The listing builds one solid part. Answer for the finished solid, in the listing's coordinates (mm). A direction names the side the tool comes from. Give positions to 0.01 mm unless a question says otherwise; leave off trailing zeros. Loops run counter-clockwise (first coordinate to the right, second up) from the corner with the lowest first, then second, coordinate; pieces in that order, holes last. Notation, with made-up numbers: (42, 49.5) - (73, 49.5) arc R27 ccw to (73, 83.5) - close; hole circle Ø2 at (56.25, -35). An arc over 180 degrees is marked (long way). Answer as CSV lines item,"result". Start each with the question number.
1) A cutting plane is placed at D-D (z = 49). Determine the outline of the cut face in (x, y) (3 decimals).
2) Find the intervals of material crossed by line 1 along Z through (x, y) = (11, -15.5) (3 decimals); line 2 along X through (y, z) = (10.5, 45.5); line 3 along Z through (x, y) = (-10, 4.5) (3 decimals), in increasing order.
3) For a pull along Z with two mould halves and no side action, classify faces 1 (the face through (-9, -9, 82.6)), 2 (the face through (19.98, -0.88, 69.71)), 3 (the face through (-9, 4, 25.425)) as pulls with the +Z half, pulls with the -Z half, needs draft (parallel to the pull), parting line crosses it, or undercut.
4) For faces 4 (the face through (0, 11.604, 42)), 5 (the face through (11.923, 3.755, 91.219)), 6 (the face through (11.923, 3.755, -8.381)), 7 (the face through (2.381, 10, 42)), determine the directions among +Z, -Z, +X, -X, +Y, -Y from which every point of the face is accessible in a straight line to the end or side of a thin tool.
5) Flat-ended cylindrical pins translate along their axes: pin 1 (1 mm diameter, centred on x = -10.5, y = 8, fed in from -Z); pin 2 (10 mm diameter, centred on x = -11.5, z = 78, fed in from +Y); pin 3 (6 mm diameter, centred on x = 13, y = -16, fed in from +Z). Find the tip coordinate at first contact, or state that the pin passes through.
6) A cutting plane is placed at C-C (x = 0). Determine the outline of the cut face in (y, z) (3 decimals), and give its area (3 significant figures).
7) A cutting plane is placed at A-A (y = 0). Determine the outline of the cut face in (x, z) (3 decimals).
8) A cutting plane is placed at B-B (x = 15.5). Determine the outline of the cut face in (y, z) (3 decimals).
```python
from build123d import *

# Parameters (mm, degrees)
SKETCH1_R           = 12.5
BOSS_EXTRUDE1_DEPTH = 17
SKETCH2_R           = 20
BOSS_EXTRUDE2_DEPTH = 25.425
SKETCH3_R           = 9.525
BOSS_EXTRUDE3_DEPTH = 31.75
SKETCH9_W           = 4.7625
SKETCH9_H           = 2.38125
BOSS_EXTRUDE6_DEPTH = 31.75
SKETCH4_R           = 20
BOSS_EXTRUDE4_DEPTH = 25.425
BOSS_EXTRUDE5_START = 17
SKETCH5_R           = 12.5
BOSS_EXTRUDE5_DEPTH = 17


with BuildPart() as part:
    # Sketch1 → Boss-Extrude1 (new body)
    with BuildSketch(Plane.XY):
        Circle(SKETCH1_R)
    extrude(amount=-BOSS_EXTRUDE1_DEPTH)

    # Sketch2 → Boss-Extrude2 (add)
    with BuildSketch(Plane.XY):
        with Locations(Location((0, 0, 0), (0, 0, 180))):
            Circle(SKETCH2_R)
    extrude(amount=BOSS_EXTRUDE2_DEPTH)

    # Sketch3 → Boss-Extrude3 (add)
    with BuildSketch(Plane.XY.offset(25.425)):
        Circle(SKETCH3_R)
    extrude(amount=BOSS_EXTRUDE3_DEPTH)

    # Sketch9 → Boss-Extrude6 (add)
    with BuildSketch(Plane.XY.offset(57.175)):
        with Locations((0, 10.413166593)):
            Rectangle(SKETCH9_W, SKETCH9_H)
    extrude(amount=-BOSS_EXTRUDE6_DEPTH)

    # Sketch4 → Boss-Extrude4 (add)
    with BuildSketch(Plane.XY.offset(57.175)):
        with Locations(Location((0, 0, 0), (0, 0, 180))):
            Circle(SKETCH4_R)
    extrude(amount=BOSS_EXTRUDE4_DEPTH)

    # Sketch5 → Boss-Extrude5 (add)
    with BuildSketch(Plane.XY.offset(82.6).offset(BOSS_EXTRUDE5_START)):
        Circle(SKETCH5_R)
    extrude(amount=-BOSS_EXTRUDE5_DEPTH)


solid = part.part
```
Ans:
1,outline,"(-2.381, 9.223) arc R9.525 ccw (long way) to (2.381, 9.223) - (2.381, 11.604) - (-2.381, 11.604) - close"
2,line 1,"0 to 25.425, 57.175 to 82.6"
2,line 2,"-2.38 to 2.38"
2,line 3,"-17 to 25.425, 57.175 to 99.6"
3,face 1,"pulls with the +Z half"
3,face 2,"needs draft"
3,face 3,"undercut"
4,face 4,"+X, -X, +Y"
4,face 5,"+Z"
4,face 6,"-Z"
4,face 7,"+X, +Y"
5,pin 1,"z = 0"
5,pin 2,"y = 18.91"
5,pin 3,"z = 82.6"
6,outline,"(-20, 0) - (-12.5, 0) - (-12.5, -17) - (12.5, -17) - (12.5, 0) - (20, 0) - (20, 25.425) - (11.604, 25.425) - (11.604, 57.175) - (20, 57.175) - (20, 82.6) - (12.5, 82.6) - (12.5, 99.6) - (-12.5, 99.6) - (-12.5, 82.6) - (-20, 82.6) - (-20, 57.175) - (-9.525, 57.175) - (-9.525, 25.425) - (-20, 25.425) - close"
6,area,"3,550 mm2"
7,outline,"(-20, 0) - (-12.5, 0) - (-12.5, -17) - (12.5, -17) - (12.5, 0) - (20, 0) - (20, 25.425) - (9.525, 25.425) - (9.525, 57.175) - (20, 57.175) - (20, 82.6) - (12.5, 82.6) - (12.5, 99.6) - (-12.5, 99.6) - (-12.5, 82.6) - (-20, 82.6) - (-20, 57.175) - (-9.525, 57.175) - (-9.525, 25.425) - (-20, 25.425) - close"
8,outline,"(-12.639, 0) - (12.639, 0) - (12.639, 25.425) - (-12.639, 25.425) - close; (-12.639, 57.175) - (12.639, 57.175) - (12.639, 82.6) - (-12.639, 82.6) - close"
